Check sheet for the modelled part. Datum: model origin and axes. Units: mm. A direction names the side the tool comes from. Give positions to 0.01 mm unless a question says otherwise; leave off trailing zeros. Order: outer loops, then holes, each group sorted by start corner. A loop starts at its lowest first (then second) coordinate and runs counter-clockwise, first axis right, second up. Notation, with made-up numbers: M -3,-28.5 L 31,-28.5 A7 ccw 31,-20.5 Z; hole C 36,-13 d3. An arc over 180 degrees is marked long. Answer in a Markdown table with one row per item. Add a question column.
Autodesk Fusion 360 part; units mm, degrees
sketch "Sketch1" plane through (0, 0, 0) normal (0, 0, 1) x (1, 0, 0)
  line L0 (41.26, -53.9475) -> (-23.8891, -34.972)
  arc A0 (41.26, -53.9475) -> (-52.9571, 42.103) centre (-23.9263, -23.6549) ccw
  line L1 (-49.1844, 40.1007) -> (-34.6167, -16.2167)
  line L2 (-34.6167, -16.2167) -> (-20.6815, -2.1702)
  line L3 (-3.8871, -18.8317) -> (-18.0593, -33.1169)
  line L4 (-18.0593, -33.1169) -> (39.4437, -49.8653)
  arc A1 (23.8726, 25.5184) -> (-49.1844, 40.1007) centre (-23.9263, -23.6549) ccw
  line L5 (23.8726, 25.5184) -> (-12.7212, -10.0675)
  line L6 (25.8056, 23.5625) -> (-10.9878, -11.7872)
  arc A2 (39.4437, -49.8653) -> (25.8056, 23.5625) centre (-23.9263, -23.6549) ccw
  line L7 (23.8726, 25.5184) -> (28.5034, 25.5184) construction
  line L8 (-20.6815, -2.1702) -> (-12.7212, -10.0675)
  line L9 (-10.9878, -11.7872) -> (-3.8871, -18.8317)
  line L10 (-36.4169, -21.8399) -> (-29.7834, -15.1535)
  line L11 (-20.9093, -6.2086) -> (-8.0298, -18.9862)
  line L12 (-16.9038, -27.9311) -> (-23.8891, -34.972)
  line L13 (-52.9571, 42.103) -> (-36.4169, -21.8399)
  line L14 (-8.0298, -18.9862) -> (-14.0867, -25.0914)
  line L15 (-14.0867, -25.0914) -> (-15.5065, -23.6828)
  line L16 (-15.5065, -23.6828) -> (-18.3237, -26.5225)
  line L17 (-18.3237, -26.5225) -> (-16.9038, -27.9311)
  line L18 (-26.9662, -12.3138) -> (-20.9093, -6.2086)
  line L19 (-26.9662, -12.3138) -> (-25.5464, -13.7224)
  line L20 (-25.5464, -13.7224) -> (-28.3636, -16.562)
  line L21 (-28.3636, -16.562) -> (-29.7834, -15.1535)
  line L22 (-18.3237, -26.5225) -> (-25.3088, -33.5634)
  line L23 (-25.3088, -33.5634) -> (-23.8891, -34.972)
  line L24 (-36.4169, -21.8399) -> (-34.9971, -23.2485)
  line L25 (-34.9971, -23.2485) -> (-28.3636, -16.562)
  dimension "d4" = 2
  dimension "d5" = 4
  dimension "d6" = 2
  dimension "d7" = 4
  dimension "d8" = 9.918
  dimension "d9" = 2
extrude "Extrude1" add sketch "Sketch1" along normal blind 4.7
sketch "Sketch2" plane through (0, 0, 4.7) normal (0, 0, 1) x (-1, 0, 0)
  arc A0 (-23.8726, -25.5184) -> (49.1844, -40.1007) centre (23.9263, 23.6549) ccw
  line L0 (-23.8726, -25.5184) -> (12.7212, 10.0675)
  line L1 (12.7212, 10.0675) -> (20.6815, 2.1702)
  line L2 (20.6815, 2.1702) -> (34.6167, 16.2167)
  line L3 (34.6167, 16.2167) -> (49.1844, -40.1007)
  line L4 (3.8871, 18.8317) -> (10.9878, 11.7872)
  line L5 (10.9878, 11.7872) -> (-25.8056, -23.5625)
  arc A1 (-39.4437, 49.8653) -> (-25.8056, -23.5625) centre (23.9263, 23.6549) ccw
  line L6 (-39.4437, 49.8653) -> (18.0593, 33.1169)
  line L7 (18.0593, 33.1169) -> (3.8871, 18.8317)
  arc A2 (-41.26, 53.9475) -> (52.9571, -42.103) centre (23.9263, 23.6549) ccw
  line L8 (52.9571, -42.103) -> (36.4169, 21.8399)
  line L9 (36.4169, 21.8399) -> (34.9971, 23.2485)
  line L10 (34.9971, 23.2485) -> (25.5464, 13.7224)
  line L11 (25.5464, 13.7224) -> (26.9662, 12.3138)
  line L12 (26.9662, 12.3138) -> (20.9093, 6.2086)
  line L13 (20.9093, 6.2086) -> (8.0298, 18.9862)
  line L14 (8.0298, 18.9862) -> (14.0867, 25.0914)
  line L15 (14.0867, 25.0914) -> (15.5065, 23.6828)
  line L16 (15.5065, 23.6828) -> (25.3088, 33.5634)
  line L17 (25.3088, 33.5634) -> (23.8891, 34.972)
  line L18 (23.8891, 34.972) -> (-41.26, 53.9475)
  line L19 (16.9038, 27.9311) -> (18.3237, 26.5225)
  line L20 (16.9038, 27.9311) -> (23.8891, 34.972)
  line L21 (36.4169, 21.8399) -> (29.7834, 15.1535)
  line L22 (29.7834, 15.1535) -> (28.3636, 16.562)
  dimension "d12" = 4
  dimension "d13" = 4
extrude "Extrude2" add sketch "Sketch2" along normal blind 2.8 contours L16 L17 L19 L20 | L9 L10 L21 L22
Q1. Cross-section at B-B (y = 14). Record the boundary of the cut face in (x, z).
Q2. Tool access check on faces 4 (the flat face through (-44.803, 10.579, 2.317)), 5 (the flat face through (-14.56, -12.51, 2.32)), 6 (the flat face through (-20.348, -31.402, 6.08)). Record the directions out of +Z, -Z, +X, -X, +Y, -Y that give a thin tool (end or side, any length) a straight path to the whole face; none if there is none.
Q3. Cross-section at C-C (x = 4). Record the boundary of the cut face in (y, z), and give its area (3 significant figures).
Q4. Draft check along X on faces 1 (the flat face through (-3, -3, 0)), 2 (the flat face through (9.141, -44.593, 2.317)), 3 (the flat face through (-16.76, -6.06, 2.32)). Enter one of: pulls with the +X half, pulls with the -X half, needs draft (parallel to the pull), parting line crosses it, or undercut.
Q5. Cross-section at A-A (z = 6). Record the boundary of the cut face in (x, y).
Q6. Go/stop test with flat-tipped pins: pin 1 (4 mm diameter, centred on y = -8, z = 6, fed in from +X); pin 2 (3 mm diameter, centred on x = 30.5, z = 3.5, fed in from -Y); pin 3 (4 mm diameter, centred on x = -39, y = -10, fed in from +Z). Record where each tip stops, or that it passes through.
Q7. Thickness scan on probe 1 along X at (y, z) = (17.5, 3.5); probe 2 along Y at (x, z) = (15.5, 4.25); probe 3 along Y at (x, z) = (-7.5, 4). Record the ranges inside material, lowest first.
Q8. Cross-section at D-D (x = 36). Record the boundary of the cut face in (y, z).
Values follow:
| question | item | result |
|---|---|---|
| 1 | outline | M -45.69,0 L -42.43,0 L -42.43,4.7 L -45.69,4.7 Z; M 12.03,0 L 15.85,0 L 15.85,4.7 L 12.03,4.7 Z; M 33.39,0 L 37.3,0 L 37.3,4.7 L 33.39,4.7 Z |
| 2 | face 4 | +Z, -Z, -X, -Y |
| 2 | face 5 | +Z, -Z |
| 2 | face 6 | +Z, +X, -Y |
| 3 | outline | M -43.1,0 L -39.54,0 L -39.54,4.7 L -43.1,4.7 Z; M 2.61,0 L 6.19,0 L 6.19,4.7 L 2.61,4.7 Z; M 38.98,0 L 42.58,0 L 42.58,4.7 L 38.98,4.7 Z |
| 3 | area | 50.5 mm² |
| 4 | face 1 | needs draft |
| 4 | face 2 | pulls with the -X half |
| 4 | face 3 | undercut |
| 5 | outline | M -36.42,-21.84 L -35,-23.25 L -28.36,-16.56 L -29.78,-15.15 Z; M -25.31,-33.56 L -23.89,-34.97 L -16.9,-27.93 L -18.32,-26.52 Z |
| 6 | pin 1 | x = 46.55 |
| 6 | pin 2 | y = -51.25 |
| 6 | pin 3 | z = 4.7 |
| 7 | probe 1 | -46.59 to -43.34, 15.63 to 19.5, 30.93 to 35.01 |
| 7 | probe 2 | -46.44 to -42.89, 13.66 to 17.38, 32.45 to 36.45 |
| 7 | probe 3 | -39.75 to -36.19, -22.47 to -15.25, -8.44 to -4.99, 42.93 to 46.32 |
| 8 | outline | M -52.42,0 L -48.86,0 L -48.86,4.7 L -52.42,4.7 Z; M 9.69,0 L 16.04,0 L 16.04,4.7 L 9.69,4.7 Z |
